```python
from build123d import *

# Parameters (mm, degrees)
SKETCH1_R           = 4
SKETCH1_R_2         = 2
BOSS_EXTRUDE1_DEPTH = 5
FILLET1_R           = 4
FILLET2_R           = 3
FILLET3_R           = 3


with BuildPart() as part:
    # Sketch1 → Boss-Extrude1 (new body)
    with BuildSketch(Plane(origin=(0, 0, 0), x_dir=(1, 0, 0), z_dir=(0, 1, 0))):
        with BuildLine():
            Line((-16, 33.943656531), (-16, 32.943656531))
            ThreePointArc((-16, 32.943656531), (-11.633307653, 18.521451429), (0, 8.943656531))
            ThreePointArc((0, 8.943656531), (11.633307653, 18.521451429), (16, 32.943656531))
            Line((16, 32.943656531), (16, 33.943656531))
            Line((16, 33.943656531), (18, 33.943656531))
            ThreePointArc((18, 33.943656531), (22.110006153, 24.491379681), (23.514801823, 14.280393571))
            Line((23.514801823, 14.280393571), (23.514801823, 13.884283426))
            ThreePointArc((23.514801823, 13.884283426), (25.450700755, 11.237241369), (28.138825911, 9.35880599))
            ThreePointArc((28.138825911, 9.35880599), (31.417131183, 2.664821909), (25.64875, -2.055611002))
            ThreePointArc((25.64875, -2.055611002), (23.370974699, -2.355136602), (21.221666667, -3.166586471))
            ThreePointArc((21.221666667, -3.166586471), (16.57103717, -3.995601441), (12.263497378, -2.056343469))
            Line((12.263497378, -2.056343469), (-12.263497378, -2.056343469))
            ThreePointArc((-12.263497378, -2.056343469), (-23.233209016, -1.691762031), (-23.514801823, 9.280393571))
            Line((-23.514801823, 9.280393571), (-23.514801823, 14.280393571))
            ThreePointArc((-23.514801823, 14.280393571), (-22.110006153, 24.491379681), (-18, 33.943656531))
            Line((-18, 33.943656531), (-16, 33.943656531))
        make_face()
        with Locations(Location((17.555, 3.943656531, 0), (0, 0, 270))):
            Circle(SKETCH1_R, mode=Mode.SUBTRACT)
        with Locations(Location((25.555, 3.943656531, 0), (0, 0, 270))):
            Circle(SKETCH1_R_2, mode=Mode.SUBTRACT)
        with Locations(Location((-1.445, 3.943656531, 0), (0, 0, 270))):
            Circle(SKETCH1_R_2, mode=Mode.SUBTRACT)
        with BuildLine():
            Line((-19.585, 5.943656531), (-15.585, 5.943656531))
            ThreePointArc((-15.585, 5.943656531), (-13.585, 3.943656531), (-15.585, 1.943656531))
            Line((-15.585, 1.943656531), (-19.585, 1.943656531))
            ThreePointArc((-19.585, 1.943656531), (-21.585, 3.943656531), (-19.585, 5.943656531))
        make_face(mode=Mode.SUBTRACT)
    extrude(amount=BOSS_EXTRUDE1_DEPTH)

    # Fillet1
    fillet1_edges = [part.edges().sort_by_distance(p)[0] for p in [
        (0, 2.5, -8.943656531),
    ]]
    fillet(fillet1_edges, radius=FILLET1_R)

    # Fillet2
    # the kernel refuses this fillet: 3 mm, written as the material it takes off along each edge
    with BuildSketch(Plane(origin=(-16, -6.644712065, -33.943656531), x_dir=(0.019894609369720675, 0, 0.999802082673379), z_dir=(0, 1, 0))) as fillet2_piece_1:
        with BuildLine():
            CenterArc((2.789518237, -2.997110716), FILLET2_R, 92.514820362, 68.064461233)
            Line((-0.039789219, -1.999604165), (-0.322719964, -1.89985351))
            ThreePointArc((-0.322719964, -1.89985351), (-0.319835234, -0.9938337), (-0.299940625, 0.005968383))
            Line((-0.299940625, 0.005968383), (0.005968383, 0.299940625))
            ThreePointArc((0.005968383, 0.299940625), (1.005770465, 0.280046015), (2.644721485, 0.299711072))
            Line((2.644721485, 0.299711072), (2.657884826, 0))
        make_face()
    extrude(amount=18.289424129, mode=Mode.SUBTRACT)

    # Fillet3
    # the kernel refuses this fillet: 3 mm, written as the material it takes off along each edge
    with BuildSketch(Plane(origin=(16, -6.644712065, -33.943656531), x_dir=(1, 0, 0), z_dir=(0, 1, 0))) as fillet3_piece_1:
        with BuildLine():
            CenterArc((2.94102116, -2.84859249), FILLET3_R, 108.280766047, 68.064461233)
            Line((-0.05287758, -2.657358784), (-0.352267454, -2.638235414))
            ThreePointArc((-0.352267454, -2.638235414), (-0.3, -1), (-0.3, 0))
            Line((-0.3, 0), (0, 0.3))
            ThreePointArc((0, 0.3), (1, 0.3), (1.905897884, 0.284859249))
            Line((1.905897884, 0.284859249), (2, 0))
        make_face()
    extrude(amount=18.289424129, mode=Mode.SUBTRACT)


solid = part.part
```
Design review of the part built by this model. Coordinates are the model's own, in mm. A direction names the side the tool comes from. Round coordinates to 2 decimals unless told otherwise and drop trailing zeros. Write each loop counter-clockwise with the first axis right and the second up, starting at its lowest first coordinate (ties: lowest second). Pieces come first, ordered by that corner, then holes. Notation, with made-up numbers: (46.5, -30) -> (73.5, -30) arc R21 cw to (73.5, -2) -> close; hole circle Ø9 at (-34.75, 0.5). An arc over 180 degrees is marked (long way). Write item = value, one per line. Start each with the question number.
1) Take a section at C-C, the plane x = 13. State the section outline as (y, z) points, plus the area to 3 significant figures.
2) Take a section at B-B, the plane x = -21. State the section outline as (y, z) points.
3) Clearance check with flat-ended pins moving along their axes: pin 1 (1.5 mm diameter, centred on y = 4, z = -2.5, fed in from -X); pin 2 (1.5 mm diameter, centred on y = 3.5, z = -10.5, fed in from -X); pin 3 (1.2 mm diameter, centred on x = -17, y = 2.5, fed in from -Z). State where each tip first meets the part, or that it passes through.
4) Tool access review of faces 5 (the face through (16.582, 2.465, -32.949)), 6 (the face through (-21.585, 2.465, -3.9)), 7 (the face through (16.6, 2.5, 4)), 8 (the face through (-23.515, 2, -12)): name each direction out of +Z, -Z, +X, -X, +Y, -Y from which nothing blocks a thin tool from reaching the whole face with its end or side.
5) Take a section at A-A, the plane z = -1. State the section outline as (x, y) points.
6) Mouldability with a two-part tool opening along X and no side actions: class faces 1 (the face through (3, 5, -7)), 2 (the face through (0, 2, 2.056)), 3 (the face through (23.402, 2.465, 2.347)), 4 (the face through (-11.83, 2.46, -18.82)) as +X half, -X half, draft (parallel to the pull), parting line (faces both ways), or undercut.
7) Wall thickness on probe 1 along X at (y, z) = (3.65, -5); probe 2 along Z at (x, y) = (14, 2.05); probe 3 along X at (y, z) = (1.5, -24): over which ranges is each line inside the solid? List them lowest first. Write a range as from..to.
8) Take a section at D-D, the plane y = 3.15. Count the separate pieces of the cut face and the enclosed holes in it, plus the area to 3 significant figures.
Results list:
q1.outline = (0, -20.82) -> (5, -20.82) -> (5, 2.63) -> (0, 2.63) -> close
q1.area = 117 mm²
q2.outline = (0, -27.84) -> (5, -27.84) -> (5, -5.36) -> (0, -5.36) -> close; (0, -2.53) -> (5, -2.53) -> (5, 3.28) -> (0, 3.28) -> close
q3.pin_1 = -25.52
q3.pin_2 = -23.51
q3.pin_3 = -33.78
q4.face_5 = -Z, +Y, -Y
q4.face_6 = +Y, -Y
q4.face_7 = +Z, +Y, -Y
q4.face_8 = -Z, -X, +Y, -Y
q5.outline = (-24.99, 0) -> (14.85, 0) -> (14.85, 5) -> (-24.99, 5) -> close; (20.26, 0) -> (30.78, 0) -> (30.78, 5) -> (20.26, 5) -> close
q6.face_1 = draft
q6.face_2 = undercut
q6.face_3 = +X half
q6.face_4 = undercut
q7.probe_1 = -25.48..-21.28, -13.89..-3.14, 0.25..13.7, 21.41..23.86, 27.25..31.46
q7.probe_2 = -22.94..-5.78, -2.11..3.22
q7.probe_3 = -22.24..-14.41, 14.41..22.24
q8.separate_pieces = 1
q8.enclosed_holes = 4
q8.area = 1,060 mm²
